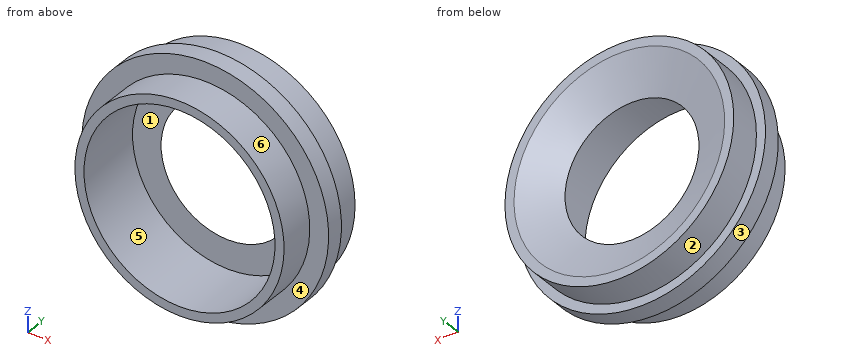
Autodesk Inventor part; units mm, degrees
ref_plane "Work Plane4" through (0, -133.7486, -73.152) normal (-1, 0, 0) x (0, 0, 1)
ref_plane "Work Plane3" through (0, -133.7486, -73.152) normal (-1, 0, 0) x (0, 0, 1)
ref_plane "Work Plane2" through (0, 9.93, 0) normal (0, -1, 0) x (1, 0, 0)
sketch "Sketch2" plane through (0, 0, 0) normal (0, 1, 0) x (-1, 0, 0)
  line L0 (0, -114.5678) -> (107.9834, -114.5678)
  line L1 (107.9834, -114.5678) -> (107.9834, 108.3126)
  line L2 (107.9834, 108.3126) -> (0, 108.3126)
  line L3 (0, 108.3126) -> (0, -114.5678)
  point P0 (0, 0)
extrude "Extrusion1" [suppressed]
ref_plane "Work Plane4" through (0, -133.7486, -73.152) normal (-1, 0, 0) x (0, 0, 1)
sketch "Sketch3" plane through (0, -133.7486, -73.152) normal (-1, 0, 0) x (0, 0, 1)
  line L0 (6.35, 143.6785) -> (6.35, 121.0486)
  line L1 (6.35, 121.0486) -> (6.35, 95.6486)
  line L2 (0, 95.6486) -> (6.35, 95.6486)
  line L3 (0, 121.0486) -> (-13.208, 121.0486)
  line L4 (-13.208, 121.0486) -> (-13.208, 133.7486)
  line L5 (-13.208, 121.0486) -> (-13.208, 133.7486)
  line L6 (-13.208, 133.7486) -> (-6.858, 133.7486)
  line L7 (-6.858, 133.7486) -> (-6.858, 156.1875)
  line L8 (-0.508, 156.1875) -> (26.3176, 143.6785)
  line L9 (-6.858, 156.1875) -> (-0.508, 156.1875)
  line L10 (-0.508, 156.1875) -> (26.3176, 143.6785)
  line L11 (12.7, 143.6785) -> (26.3176, 143.6785)
  line L12 (6.35, 143.6785) -> (12.7, 143.6785)
  line L13 (314.1117, 153.1152) -> (314.1117, 130.4853)
  line L14 (314.1117, 130.4853) -> (314.1117, 105.0853)
  line L15 (307.7617, 105.0853) -> (314.1117, 105.0853)
  line L16 (307.7617, 130.4853) -> (294.5537, 130.4853)
  line L17 (294.5537, 130.4853) -> (294.5537, 143.1853)
  line L18 (294.5537, 143.1853) -> (300.9037, 143.1853)
  line L19 (300.9037, 143.1853) -> (300.9037, 165.6242)
  line L20 (307.2537, 165.6242) -> (334.0793, 153.1152)
  line L21 (300.9037, 165.6242) -> (307.2537, 165.6242)
  line L22 (320.4617, 153.1152) -> (334.0793, 153.1152)
  line L23 (314.1117, 153.1152) -> (320.4617, 153.1152)
  line L24 (334.0793, 153.1152) -> (380.9169, 153.1152) construction
  line L25 (380.9169, 153.1152) -> (380.9169, 203.9215) construction
  line L26 (307.7617, 130.4853) -> (307.7617, 105.0853)
  line L27 (0, 121.0486) -> (0, 95.6486)
  line L28 (0, 0) -> (0, 121.0486)
  point P0 (73.152, 133.7486)
  dimension "d32" = 6.35
  dimension "d34" = 6.35
  dimension "d35" = 46.8376
revolve "Revolution3" add sketch "Sketch3" angle 360 about axis through (0, 19.3666, 307.7649) along (0, 1, 0) contours L13 L14 L15 L26 L16 L17 L18 L19 L21 L20 L22 L23
ref_plane "Work Plane3" through (0, -133.7486, -73.152) normal (-1, 0, 0) x (0, 0, 1)
sketch "Sketch6" plane through (0, -133.7486, -73.152) normal (-1, 0, 0) x (0, 0, 1)
  line L0 (0, 121.0486) -> (0, 95.6486)
  line L1 (0, 95.6486) -> (6.35, 95.6486)
  line L2 (0, 121.0486) -> (-13.208, 121.0486)
  line L3 (-13.208, 121.0486) -> (-13.208, 133.7486)
  line L4 (-13.208, 121.0486) -> (-13.208, 133.7486)
  line L5 (-13.208, 133.7486) -> (-6.858, 133.7486)
  line L6 (-6.858, 133.7486) -> (-6.858, 156.1875)
  line L7 (-0.508, 156.1875) -> (26.3176, 143.6785)
  line L8 (-6.858, 156.1875) -> (-0.508, 156.1875)
  line L9 (-0.508, 156.1875) -> (26.3176, 143.6785)
  line L10 (6.35, 95.6486) -> (6.35, 143.68)
  line L11 (6.35, 143.68) -> (26.3176, 143.6785)
  line L12 (26.3176, 143.6785) -> (92.5608, 143.6785) construction
  line L13 (73.152, 133.7486) -> (73.152, 183.9478) construction
  line L14 (119.9864, 143.6785) -> (26.3176, 143.6785) construction
  line L15 (26.3176, 143.6785) -> (73.152, 143.6785) construction
  dimension "d37" = 25.4
  dimension "d38" = 6.35
  dimension "d39" = 6.35
  dimension "d40" = 48.0314
revolve "Revolution4" cut sketch "Sketch6" angle 360 about axis through (0, 0, 0) along (0, 1, 0)
ref_plane "Work Plane2" through (0, 9.93, 0) normal (0, -1, 0) x (1, 0, 0)
sketch "Sketch7" plane through (0, 9.93, 0) normal (0, -1, 0) x (1, 0, 0)
  point P0 (0, 0)
ref_plane "Work Plane1" through (0, 9.93, 0) normal (0, -1, 0) x (1, 0, 0)
sketch "Sketch8" plane through (0, 9.93, 0) normal (0, -1, 0) x (1, 0, 0)
  point P0 (0, 0)
ref_plane "Work Plane5" through (0, 9.93, 0) normal (0, -1, 0) x (1, 0, 0)
sketch "Sketch9" plane through (0, 9.93, 0) normal (0, -1, 0) x (1, 0, 0)
  circle A0 centre (0, 0) radius 60.7129
extrude "Extrusion2" cut sketch "Sketch9" along normal mid plane 25.4
properties part number "part 2 cap of Phenolic Master Sketch" material "Phenolic Resin"
Could you check a few things on this model? Use its own coordinates, in mm. Face numbers are marked on the shaded views. A direction names the side the tool comes from. Round coordinates to 2 decimals unless told otherwise and drop trailing zeros. Loops run counter-clockwise (first coordinate to the right, second up) from the corner with the lowest first, then second, coordinate; pieces in that order, holes last. Notation, with made-up numbers: M 20,-27.75 L 43,-27.75 A32 cw 43,6.25 Z; hole C 62,77 d9. An arc over 180 degrees is marked long. Write item = value, one per line.
1. I want a section at C-C, the plane y = 27. Write out the boundary of the cut face in (x, z), and give its area (3 significant figures).
Results below:
outline = C 0,307.76 d160.03; hole C 0,307.76 d126.41
area = 7,560 mm²
2. Which directions (+Z, -Z, +X, -X, +Y, -Y) give clear straight access to the entire face, cutting with the end or side of a thin tool? Please do the marked faces 1, 2 and 3.
Results below:
face_1 = -Y
face_2 = +Y
face_3 = +Y, -Y
3. I want a section at B-B, the plane y = 6.5. Write out the boundary of the cut face in (x, z), and give its area (3 significant figures).
Results below:
outline = C 0,307.76 d172.73; hole C 0,307.76 d133.61
area = 9,410 mm²
4. I want a section at A-A, the plane x = 0. Write out the boundary of the cut face in (y, z), and give its area (3 significant figures).
Results below:
outline = M -28.66,234.61 L -3.26,234.61 L -3.26,221.4 L 9.44,221.4 L 9.44,227.75 L 31.88,227.75 L 31.88,234.1 L 19.37,260.93 L 19.37,240.96 L -28.66,240.96 Z; M -28.66,374.57 L 19.37,374.57 L 19.37,354.6 L 31.88,381.43 L 31.88,387.78 L 9.44,387.78 L 9.44,394.13 L -3.26,394.13 L -3.26,380.92 L -28.66,380.92 Z
area = 1,580 mm²
5. Thinking about a two-plate mould opening in Z: for the marked faces 4, 5 and 6, which applies, +Z half, -Z half, draft (parallel to the pull), parting line (faces both ways), or undercut?
Results below:
face_4 = draft
face_5 = undercut
face_6 = parting line
6. Will these pins go through, and if not, where does the flat tip stop? P1, Ø1.5, axis at x = 41, y = -11, coming from the -Z side; P2, Ø8, axis at x = -39, y = -18.5, coming from the -Z side; P3, Ø3, axis at y = -16.5, z = 344.5, coming from the -X side.
Results below:
P1 = 246.68
P2 = 243.53
P3 = -64.11
7. I need wall thicknesses on probe 1 along Z at (x, y) = (1, 8); probe 2 along Z at (x, y) = (-1.5, -19.5); probe 3 along Y at (x, z) = (-63, 359.5). Which ranges of each line are inside material? Lowest first, please.
Results below:
probe_1 = 221.41 to 240.97, 374.56 to 394.12
probe_2 = 234.63 to 240.98, 374.55 to 380.9
probe_3 = -3.26 to 9.44
